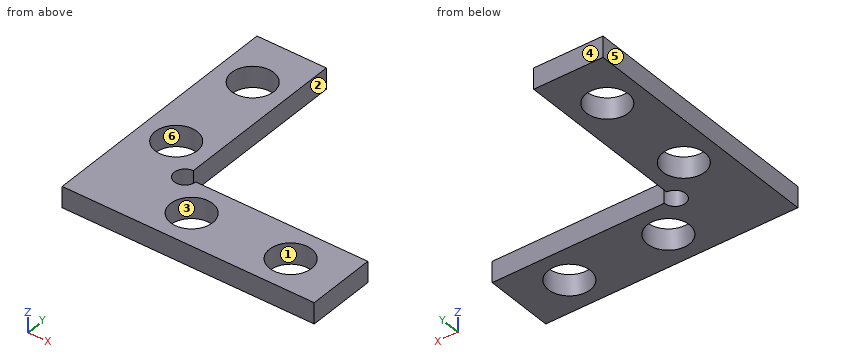
from build123d import *

# Parameters (mm, degrees)
SKETCH_1_W          = 9.9
SKETCH_1_H          = 36
EXTRUDE_1_DEPTH     = 3
SKETCH_2_W          = 36
SKETCH_2_H          = 9.9
EXTRUDE_2_DEPTH     = 3
SKETCH_3_R          = 3
CUT_EXTRUDE_1_DEPTH = 52
SKETCH_4_R          = 1.527094442
CUT_EXTRUDE_2_DEPTH = 52


with BuildPart() as part:
    # 草图1 → 凸台-拉伸1 (new body)
    with BuildSketch(Plane.XY):
        with Locations((4.95, 18)):
            Rectangle(SKETCH_1_W, SKETCH_1_H)
    extrude(amount=EXTRUDE_1_DEPTH)

    # 草图2 → 凸台-拉伸2 (add)
    with BuildSketch(Plane.XY.offset(3)):
        with Locations((18, 4.95)):
            Rectangle(SKETCH_2_W, SKETCH_2_H)
    extrude(amount=-EXTRUDE_2_DEPTH)

    # 草图3 → 切除-拉伸1 (cut, through all)
    with BuildSketch(Plane.XY.offset(3)):
        with Locations((4.95, 28.797804346)):
            Circle(SKETCH_3_R)
        with Locations((4.95, 14.661403113)):
            Circle(SKETCH_3_R)
        with Locations(Location((14.661403113, 4.95, 0), (0, 0, 180))):
            Circle(SKETCH_3_R)
        with Locations(Location((28.797804346, 4.95, 0), (0, 0, 180))):
            Circle(SKETCH_3_R)
    extrude(amount=-CUT_EXTRUDE_1_DEPTH, mode=Mode.SUBTRACT)

    # 草图4 → 切除-拉伸2 (cut, through all)
    with BuildSketch(Plane.XY.offset(3)):
        with Locations((9.9, 9.9)):
            Circle(SKETCH_4_R)
    extrude(amount=-CUT_EXTRUDE_2_DEPTH, mode=Mode.SUBTRACT)


solid = part.part
Design review of the part built by this model. Coordinates are the model's own, in mm. Face numbers are marked on the shaded views. A direction names the side the tool comes from. Round coordinates to 2 decimals unless told otherwise and drop trailing zeros. Write each loop counter-clockwise with the first axis right and the second up, starting at its lowest first coordinate (ties: lowest second). Pieces come first, ordered by that corner, then holes. Notation, with made-up numbers: (19.5, 33) - (29.5, 33) arc R17 ccw to (29.5, 58) - close; hole circle Ø9 at (-5.5, -27). An arc over 180 degrees is marked (long way). Return JSON: item names as keys, results as strings. Group by question number.
Item 1: We need section A-A on x = 4.95. Write out the cut boundary in (y, z), and give its area (3 significant figures).
Item 2: Insertion check: P1, Ø5, axis at x = 13, y = 15, coming from the -Z side; P2, Ø1.5, axis at x = 21.5, z = 1.5, coming from the +Y side; P3, Ø1, axis at y = 7, z = 2, coming from the -X side; P4, Ø1.5, axis at y = 18.5, z = 1.5, coming from the +X side. Each pin has a flat end and moves straight along its axis. Give the tip position at first contact, or say it passes through.
Item 3: The part is to be moulded in two halves that separate along Y. For the marked faces 3, 4, 5 and 6, say which applies: pulls with the +Y half, pulls with the -Y half, needs draft (parallel to the pull), parting line crosses it, or undercut.
Item 4: Machinability: for the marked faces 1 and 2, which of the approach directions +Z, -Z, +X, -X, +Y, -Y give a long, thin tool a straight path to every point of the face, cutting with its end or side? Answer none if there is none.
Item 5: We need section C-C on y = 3.5. Write out the cut boundary in (x, z), and give its area (3 significant figures).
Item 6: We need section D-D on z = 0.5. Write out the cut boundary in (x, y), and give its area (3 significant figures).
Item 7: We need section B-B on x = 28. Write out the cut boundary in (y, z), and give its area (3 significant figures).
Item 8: For probe 1 along Y at (x, z) = (5, 1.5); probe 2 along X at (y, z) = (34, 2.85), list the stretches that pass through material, from the lowest coordinate up. Write a range as [from, to].
Model answer:
{
 "1": {"outline": "(0, 0) - (11.66, 0) - (11.66, 3) - (0, 3) - close; (17.66, 0) - (25.8, 0) - (25.8, 3) - (17.66, 3) - close; (31.8, 0) - (36, 0) - (36, 3) - (31.8, 3) - close", "area": "72.0 mm²"},
 "2": {"P1": "passes through", "P2": "stops at y = 9.9", "P3": "stops at x = 0", "P4": "stops at x = 9.9"},
 "3": {"face 3": "undercut", "face 4": "pulls with the +Y half", "face 5": "needs draft", "face 6": "undercut"},
 "4": {"face 1": "+Z, -Z", "face 2": "+Z, -Z, +X, +Y"},
 "5": {"outline": "(0, 0) - (12.04, 0) - (12.04, 3) - (0, 3) - close; (17.29, 0) - (26.17, 0) - (26.17, 3) - (17.29, 3) - close; (31.42, 0) - (36, 0) - (36, 3) - (31.42, 3) - close", "area": "76.5 mm²"},
 "6": {"outline": "(0, 0) - (36, 0) - (36, 9.9) - (11.43, 9.9) arc R1.53 cw (long way) to (9.9, 11.43) - (9.9, 36) - (0, 36) - close; hole circle Ø6 at (4.95, 14.66); hole circle Ø6 at (4.95, 28.8); hole circle Ø6 at (14.66, 4.95); hole circle Ø6 at (28.8, 4.95)", "area": "496 mm²"},
 "7": {"outline": "(0, 0) - (2.06, 0) - (2.06, 3) - (0, 3) - close; (7.84, 0) - (9.9, 0) - (9.9, 3) - (7.84, 3) - close", "area": "12.3 mm²"},
 "8": {"probe 1": "y = [0, 11.66], [17.66, 25.8], [31.8, 36]", "probe 2": "x = [0, 9.9]"}
}
